```python
from build123d import *

# Parameters (mm, degrees)
SKETCH1_R           = 2.1
BOSS_EXTRUDE1_DEPTH = 2
FILLET1_R           = 1
FILLET2_R           = 1
FILLET3_R           = 1
FILLET4_R           = 1
FILLET5_R           = 1
FILLET6_R           = 1


with BuildPart() as part:
    # Sketch1 → Boss-Extrude1 (new body)
    with BuildSketch(Plane(origin=(0, 0, 0), x_dir=(1, 0, 0), z_dir=(0, 1, 0))):
        Polygon((-6.5, 0), (6.5, 0), (6.5, 5), (4, 5), (4, 29), (-4, 29), (-4, 5), (-6.5, 5), align=None)
        with Locations(Location((0, 11.1, 0), (0, 0, 270))):
            Circle(SKETCH1_R, mode=Mode.SUBTRACT)
        with Locations(Location((0, 23.5, 0), (0, 0, 270))):
            Circle(SKETCH1_R, mode=Mode.SUBTRACT)
    extrude(amount=BOSS_EXTRUDE1_DEPTH)

    # Fillet1
    fillet1_edges = [part.edges().sort_by_distance(p)[0] for p in [
        (6.5, 1, 0),
    ]]
    fillet(fillet1_edges, radius=FILLET1_R)

    # Fillet2
    fillet2_edges = [part.edges().sort_by_distance(p)[0] for p in [
        (6.5, 1, -5),
    ]]
    fillet(fillet2_edges, radius=FILLET2_R)

    # Fillet3
    fillet3_edges = [part.edges().sort_by_distance(p)[0] for p in [
        (-6.5, 1, 0),
    ]]
    fillet(fillet3_edges, radius=FILLET3_R)

    # Fillet4
    fillet4_edges = [part.edges().sort_by_distance(p)[0] for p in [
        (-6.5, 1, -5),
    ]]
    fillet(fillet4_edges, radius=FILLET4_R)

    # Fillet5
    fillet5_edges = [part.edges().sort_by_distance(p)[0] for p in [
        (-4, 1, -29),
    ]]
    fillet(fillet5_edges, radius=FILLET5_R)

    # Fillet6
    fillet6_edges = [part.edges().sort_by_distance(p)[0] for p in [
        (4, 1, -29),
    ]]
    fillet(fillet6_edges, radius=FILLET6_R)


solid = part.part
```
CAD build for the part. Positions are in the model's coordinates, mm. A direction names the side the tool comes from. Coordinates: 2 decimals unless noted, no trailing zeros. Order: outer loops, then holes, each group sorted by start corner. A loop starts at its lowest first (then second) coordinate and runs counter-clockwise, first axis right, second up.
(1) Mould opens along Z. For faces 4 (the face through (0, 1, 0)), 5 (the face through (6.215, 1.014, -4.699)), 6 (the face through (0.631, 0.986, -9.097)), 7 (the face through (4, 1, -16)) say: released by +Z, released by -Z, zero draft, split by the parting line, or undercut.
Solution:
face 4: released by +Z
face 5: released by -Z
face 6: undercut
face 7: zero draft
(2) Which spindle directions (+Z, -Z, +X, -X, +Y, -Y) get a long thin tool onto all of the face, cutting with end or side? Do faces 1 (the face through (0, 0, -15)), 2 (the face through (5, 1, -5)), 3 (the face through (-5, 1, -5)). Say none if no direction does.
Solution:
face 1: +Z, -Z, +X, -X, -Y
face 2: -Z, +X, +Y, -Y
face 3: -Z, -X, +Y, -Y
(3) Drill centre lines: L1, parallel to X at y = 1.55, z = -11.1; L2, parallel to Z at x = -1.75, y = 1.55; L3, parallel to X at y = 1.55, z = -14.75. Where is each one in solid material? Low to high.
Solution:
L1: x = -4 to -2.1, 2.1 to 4
L2: z = -29 to -24.66, -22.34 to -12.26, -9.94 to 0
L3: x = -4 to 4
(4) Saw through at D-D, the plane z = -16.25. Write the cut outline in (x, y), and give its area (3 significant figures).
Solution:
outline: (-4, 0) - (4, 0) - (4, 2) - (-4, 2) - close
area: 16.0 mm2
(5) Saw through at C-C, the plane y = 1.45. Write the cut outline in (x, z), and give its area (3 significant figures).
Solution:
outline: (-6.5, -4) arc R1 ccw to (-5.5, -5) - (-4, -5) - (-4, -28) arc R1 ccw to (-3, -29) - (3, -29) arc R1 ccw to (4, -28) - (4, -5) - (5.5, -5) arc R1 ccw to (6.5, -4) - (6.5, -1) arc R1 ccw to (5.5, 0) - (-5.5, 0) arc R1 ccw to (-6.5, -1) - close; hole circle Ø4.2 at (0, -23.5); hole circle Ø4.2 at (0, -11.1)
area: 228 mm2
(6) Saw through at B-B, the plane x = 0. Write the cut outline in (y, z), and give its area (3 significant figures).
Solution:
outline: (0, -29) - (2, -29) - (2, -25.6) - (0, -25.6) - close; (0, -21.4) - (2, -21.4) - (2, -13.2) - (0, -13.2) - close; (0, -9) - (2, -9) - (2, 0) - (0, 0) - close
area: 41.2 mm2
(7) Pin check, flat tip, straight feed: pin 1 Ø0.6 at (y, z) = (1.5, -11.5) entering from +X. Stop position of the tip, or through.
Solution:
pin 1: stops at x = 4
(8) Saw through at A-A, the plane z = -23.5. Write the cut outline in (x, y).
Solution:
outline: (-4, 0) - (-2.1, 0) - (-2.1, 2) - (-4, 2) - close; (2.1, 0) - (4, 0) - (4, 2) - (2.1, 2) - close
